from build123d import *

# Parameters (mm, degrees)
SKETCH3_W           = 15
SKETCH3_H           = 15
BOSS_EXTRUDE1_DEPTH = 3
SKETCH4_R           = 4
BOSS_EXTRUDE2_DEPTH = 5
SKETCH5_R           = 3.1
CUT_EXTRUDE1_DEPTH  = 4.5


with BuildPart() as part:
    # Sketch3 → Boss-Extrude1 (new body)
    with BuildSketch(Plane.XY):
        Rectangle(SKETCH3_W, SKETCH3_H)
    extrude(amount=BOSS_EXTRUDE1_DEPTH)

    # Sketch4 → Boss-Extrude2 (add)
    with BuildSketch(Plane.XY.offset(3)):
        Circle(SKETCH4_R)
    extrude(amount=BOSS_EXTRUDE2_DEPTH)

    # Sketch5 → Cut-Extrude1 (cut)
    with BuildSketch(Plane.XY.offset(8)):
        Circle(SKETCH5_R)
    extrude(amount=-CUT_EXTRUDE1_DEPTH, mode=Mode.SUBTRACT)


solid = part.part
CAD build for the part. Positions are in the model's coordinates, mm. A direction names the side the tool comes from. Give positions to 0.01 mm unless a question says otherwise; leave off trailing zeros. Loops run counter-clockwise (first coordinate to the right, second up) from the corner with the lowest first, then second, coordinate; pieces in that order, holes last. Notation, with made-up numbers: M 43.5,15 L 76.5,15 A20 cw 76.5,46 Z; hole C 81,-31 d1. An arc over 180 degrees is marked long. One line per question, with ' | ' between items. Start each with the question number.
1. Saw through at A-A on x = 0. Give the cut face in (y, z).
2. Flat gauge pins, fed straight in: pin 1 (1 mm diameter, centred on x = 0, z = 6.5, fed in from +Y); pin 2 (1.9 mm diameter, centred on x = -1, y = 1, fed in from +Z). Where does each tip first touch, or does it go through?
3. Two-plate mould, pull along X, no slides. Class faces 3 (the face through (7.5, 0, 1)), 4 (the face through (1.43, -2.75, 5.78)), 5 (the face through (2, -3, 8)): pulls with the +X half, pulls with the -X half, needs draft (parallel to the pull), parting line crosses it, or undercut.
4. Saw through at C-C on y = 6.75. Give the cut face in (x, z), plus the area to 3 significant figures.
5. 3-axis set-ups, long thin cutter, end or side, ignore diameter. For faces 1 (the face through (0, 0, 3.5)), 2 (the face through (0, -7.5, 1)): which of +Z, -Z, +X, -X, +Y, -Y reach the whole face in a straight line?
6. Probe L1, parallel to Y at x = 0, z = 6.1; L2, parallel to Z at x = 1, y = 0.75; L3, parallel to Z at x = 3, y = 4.75. List the from-to ranges inside material, lowest first. Write a range as from..to.
Result sheet:
1) outline: M -7.5,0 L 7.5,0 L 7.5,3 L 4,3 L 4,8 L 3.1,8 L 3.1,3.5 L -3.1,3.5 L -3.1,8 L -4,8 L -4,3 L -7.5,3 Z
2) pin 1: stops at y = 4 | pin 2: stops at z = 3.5
3) face 3: pulls with the +X half | face 4: undercut | face 5: needs draft
4) outline: M -7.5,0 L 7.5,0 L 7.5,3 L -7.5,3 Z | area: 45.0 mm^2
5) face 1: +Z | face 2: +Z, -Z, +X, -X, -Y
6) L1: y = -4..-3.1, 3.1..4 | L2: z = 0..3.5 | L3: z = 0..3
